Check sheet for the drawn part. Datum: minimum x, y, z corner. Units: mm. A direction names the side the tool comes from. Give positions to 0.01 mm unless a question says otherwise; leave off trailing zeros. Order: outer loops, then holes, each group sorted by start corner. A loop starts at its lowest first (then second) coordinate and runs counter-clockwise, first axis right, second up.
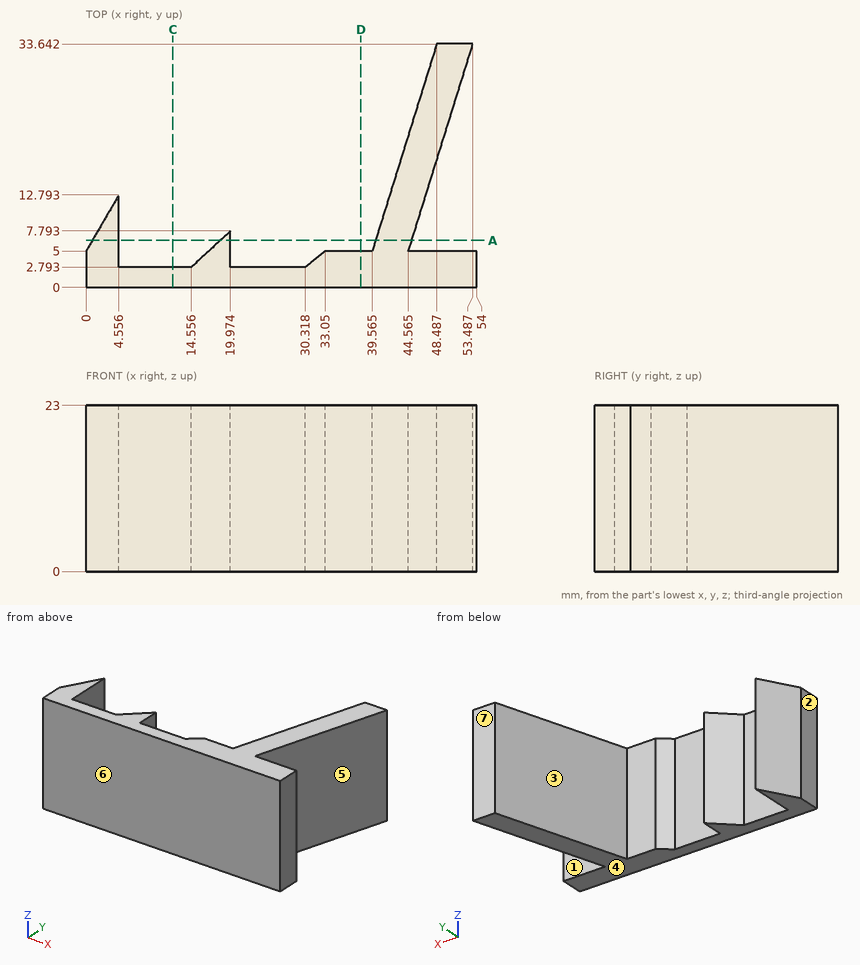
Q1. Sectioned sample at A-A, the plane y = 6.5. Record the cut outline in (x, z) (1 decimal).
Q2. Draft check along Y on the marked faces 4, 5, 6 and 7. Enter one of: pulls with the +Y half, pulls with the -Y half, needs draft (parallel to the pull), parting line crosses it, or undercut.
Q3. Sectioned sample at C-C, the plane x = 12. Record the cut outline in (y, z).
Q4. Go/stop test with flat-tipped pins: P1, Ø11.5, axis at x = 26.5, z = 15.5, coming from the +Y side (1 decimal); P2, Ø6, axis at y = 18, z = 7.5, coming from the -X side; P3, Ø2, axis at y = 8, z = 16, coming from the +X side. Record where each tip stops, or that it passes through.
Q5. Tool access check on the marked faces 1, 2 and 3. Record the directions out of +Z, -Z, +X, -X, +Y, -Y that give a thin tool (end or side, any length) a straight path to the whole face; none if there is none.
Q6. Material ranges on line 1 (Y direction, x = 24, z = 7.5); line 2 (Y direction, x = 37.5, z = 2); line 3 (X direction, y = 30, z = 1.75), recorded low to high.
Q7. Sectioned sample at D-D, the plane x = 38. Record the cut outline in (y, z).
Filled in:
1. outline: (0.9, 0) - (4.6, 0) - (4.6, 23) - (0.9, 23) - close; (18.6, 0) - (20, 0) - (20, 23) - (18.6, 23) - close; (40, 0) - (45, 0) - (45, 23) - (40, 23) - close
2. face 4: needs draft
2. face 5: undercut
2. face 6: pulls with the -Y half
2. face 7: pulls with the +Y half
3. outline: (0, 0) - (2.79, 0) - (2.79, 23) - (0, 23) - close
4. P1: stops at y = 4.4
4. P2: stops at x = 42.68
4. P3: stops at x = 45.81
5. face 1: +Z, -Z, +X
5. face 2: +Z, -Z, -X, +Y, -Y
5. face 3: +Z, -Z, +Y
6. line 1: y = 0 to 2.79
6. line 2: y = 0 to 5
6. line 3: x = 47.35 to 52.35
7. outline: (0, 0) - (5, 0) - (5, 23) - (0, 23) - close
